Here's how the part is built. I have some questions about the finished solid (model axes, mm). A direction names the side the tool comes from. Coordinates: 2 decimals unless noted, no trailing zeros. Write each loop counter-clockwise with the first axis right and the second up, starting at its lowest first coordinate (ties: lowest second). Pieces come first, ordered by that corner, then holes. Notation, with made-up numbers: (25.5, -3) -> (49.5, -3) arc R28 cw to (49.5, 27) -> close; hole circle Ø7 at (76, 57.25). An arc over 180 degrees is marked (long way). Use CSV: the item, a comma, the result in double quotes. Start each with the question number.
```python
from build123d import *

# Parameters (mm, degrees)
SKETCH_1_W          = 35.3
SKETCH_1_H          = 14.5
EXTRUDE_1_DEPTH     = 4
SKETCH_2_W          = 35.3
SKETCH_2_H          = 14.5
SKETCH_2_W_2        = 32.8
SKETCH_2_H_2        = 12
CUT_EXTRUDE_1_DEPTH = 2
SKETCH_3_W          = 29.5
SKETCH_3_H          = 11.3
EXTRUDE_2_DEPTH     = 27.5


with BuildPart() as part:
    # Эскиз1 → Бобышка-Вытянуть1 (new body)
    with BuildSketch(Plane.XY):
        Rectangle(SKETCH_1_W, SKETCH_1_H)
    extrude(amount=-EXTRUDE_1_DEPTH)

    # Эскиз2 → Вырез-Вытянуть-Тонкостенный1 (cut)
    with BuildSketch(Plane.XY):
        Rectangle(SKETCH_2_W, SKETCH_2_H)
        Rectangle(SKETCH_2_W_2, SKETCH_2_H_2, mode=Mode.SUBTRACT)
    extrude(amount=-CUT_EXTRUDE_1_DEPTH, mode=Mode.SUBTRACT)

    # Эскиз3 → Бобышка-Вытянуть2 (add)
    with BuildSketch(Plane(origin=(0, 0, -4), x_dir=(-1, 0, 0), z_dir=(0, 0, -1))):
        Rectangle(SKETCH_3_W, SKETCH_3_H)
    extrude(amount=EXTRUDE_2_DEPTH)


solid = part.part
```
Item 1: I want a section at A-A on y = 1.5. Please give me the cut outline in (x, z).
Item 2: I want a section at D-D on z = -1.5. Please give me the cut outline in (x, y).
Item 3: I'm going to push flat-ended pins straight in: pin 1 (2 mm diameter, centred on x = -14, z = -26.5, fed in from -Y); pin 2 (2 mm diameter, centred on y = -2, z = -7, fed in from -X); pin 3 (0.6 mm diameter, centred on x = -0.5, z = -0.5, fed in from +Y); pin 4 (4.5 mm diameter, centred on x = 1.5, y = -1.5, fed in from +Z). Where does each tip first touch, or does it pass through?
Item 4: I want a section at C-C on z = -12. Please give me the cut outline in (x, y).
Item 5: Which directions (+Z, -Z, +X, -X, +Y, -Y) give clear straight access to the entire face, cutting with the end or side of a thin tool? Please do faces 1 (the flat face through (0, -5.65, -18)), 2 (the flat face through (16.4, 0, -1)), 3 (the flat face through (0, 5.65, -18)), 4 (the flat face through (0, 6, -1)), 5 (the flat face through (-16.4, 0, -1)).
Item 6: If I drill on line 1 along X through (y, z) = (5, -28); line 2 along Y through (x, z) = (-11, -14.5); line 3 along Z through (x, y) = (2.5, -6.5), over which ranges is the centre line in solid material (lowest first)?
Item 7: I want a section at B-B on x = -3. Please give me the cut outline in (y, z), then the cut area to 3 significant figures.
Geometry says:
1,outline,"(-17.65, -4) -> (-14.75, -4) -> (-14.75, -31.5) -> (14.75, -31.5) -> (14.75, -4) -> (17.65, -4) -> (17.65, -2) -> (16.4, -2) -> (16.4, 0) -> (-16.4, 0) -> (-16.4, -2) -> (-17.65, -2) -> close"
2,outline,"(-16.4, -6) -> (16.4, -6) -> (16.4, 6) -> (-16.4, 6) -> close"
3,pin 1,"y = -5.65"
3,pin 2,"x = -14.75"
3,pin 3,"y = 6"
3,pin 4,"z = 0"
4,outline,"(-14.75, -5.65) -> (14.75, -5.65) -> (14.75, 5.65) -> (-14.75, 5.65) -> close"
5,face 1,"-Z, +X, -X, -Y"
5,face 2,"+Z, +X, +Y, -Y"
5,face 3,"-Z, +X, -X, +Y"
5,face 4,"+Z, +X, -X, +Y"
5,face 5,"+Z, -X, +Y, -Y"
6,line 1,"-14.75 to 14.75"
6,line 2,"-5.65 to 5.65"
6,line 3,"-4 to -2"
7,outline,"(-7.25, -4) -> (-5.65, -4) -> (-5.65, -31.5) -> (5.65, -31.5) -> (5.65, -4) -> (7.25, -4) -> (7.25, -2) -> (6, -2) -> (6, 0) -> (-6, 0) -> (-6, -2) -> (-7.25, -2) -> close"
7,area,"364 mm2"
